```python
from build123d import *

# Parameters (mm, degrees)
F0_W     = 30
F0_H     = 50
F1_DEPTH = 5
F2_W     = 6
F2_H     = 50
F2_W_2   = 7
F3_DEPTH = 5


with BuildPart() as f1:
    # F0 (on Top) → F1 (new body)
    with BuildSketch(Plane.XY):
        with Locations((15, 25)):
            Rectangle(F0_W, F0_H)
    extrude(amount=F1_DEPTH)

    # F2 (on face) → F3 (join)
    with BuildSketch(Plane.XY.offset(5)):
        with Locations((3, 25)):
            Rectangle(F2_W, F2_H)
        with Locations((15, 25)):
            Rectangle(F2_W_2, F2_H)
        with Locations((27, 25)):
            Rectangle(F2_W, F2_H)
    extrude(amount=F3_DEPTH)


solid = f1.part
```
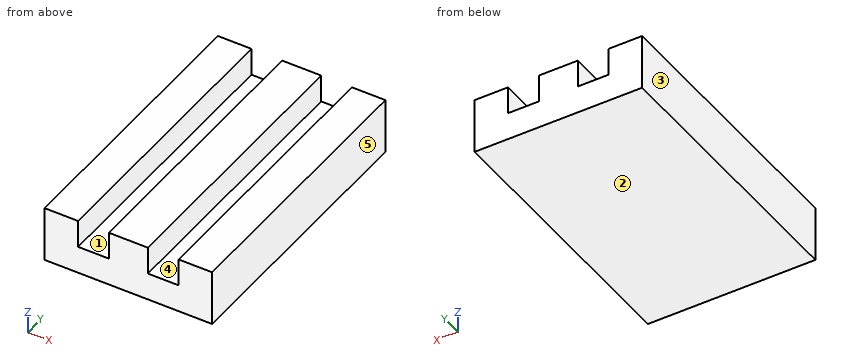
Check sheet for the modelled part. Datum: model origin and axes. Units: mm. Face numbers are marked on the shaded views. A direction names the side the tool comes from. Coordinates: 2 decimals unless noted, no trailing zeros. Write each loop counter-clockwise with the first axis right and the second up, starting at its lowest first coordinate (ties: lowest second). Pieces come first, ordered by that corner, then holes. Notation, with made-up numbers: M 52,68.5 L 65,68.5 A20 cw 65,97.5 Z; hole C 19,-5.5 d4. An arc over 180 degrees is marked long. Write item = value, one per line. Start each with the question number.
1. Sectioned sample at B-B (y = 36). Record the cut outline in (x, z).
2. Tool access check on the marked faces 4 and 5. Record the directions out of +Z, -Z, +X, -X, +Y, -Y that give a thin tool (end or side, any length) a straight path to the whole face; none if there is none.
3. Mould release check, pull along X, two halves, no side actions. Record for the marked faces 1, 2 and 3: pulls with the +X half, pulls with the -X half, needs draft (parallel to the pull), parting line crosses it, or undercut.
4. Sectioned sample at C-C (x = 7). Record the cut outline in (y, z), then the cut area to 3 significant figures.
5. Thickness scan on probe 1 along X at (y, z) = (32, 6.5); probe 2 along Z at (x, y) = (21.5, 35). Record the ranges inside material, lowest first.
6. Sectioned sample at A-A (z = 7.5). Record the cut outline in (x, y), then the cut area to 3 significant figures.
7. Go/stop test with flat-tipped pins: pin 1 (6 mm diameter, centred on y = 12, z = 7, fed in from -X); pin 2 (4.5 mm diameter, centred on x = 21, y = 15.5, fed in from +Z). Record where each tip stops, or that it passes through.
The answers:
q1.outline = M 0,0 L 30,0 L 30,10 L 24,10 L 24,5 L 18.5,5 L 18.5,10 L 11.5,10 L 11.5,5 L 6,5 L 6,10 L 0,10 Z
q2.face_4 = +Z, +Y, -Y
q2.face_5 = +Z, -Z, +X, +Y, -Y
q3.face_1 = undercut
q3.face_2 = needs draft
q3.face_3 = pulls with the -X half
q4.outline = M 0,0 L 50,0 L 50,5 L 0,5 Z
q4.area = 250 mm²
q5.probe_1 = 0 to 6, 11.5 to 18.5, 24 to 30
q5.probe_2 = 0 to 5
q6.outline = M 0,0 L 6,0 L 6,50 L 0,50 Z; M 11.5,0 L 18.5,0 L 18.5,50 L 11.5,50 Z; M 24,0 L 30,0 L 30,50 L 24,50 Z
q6.area = 950 mm²
q7.pin_1 = 0
q7.pin_2 = 5
